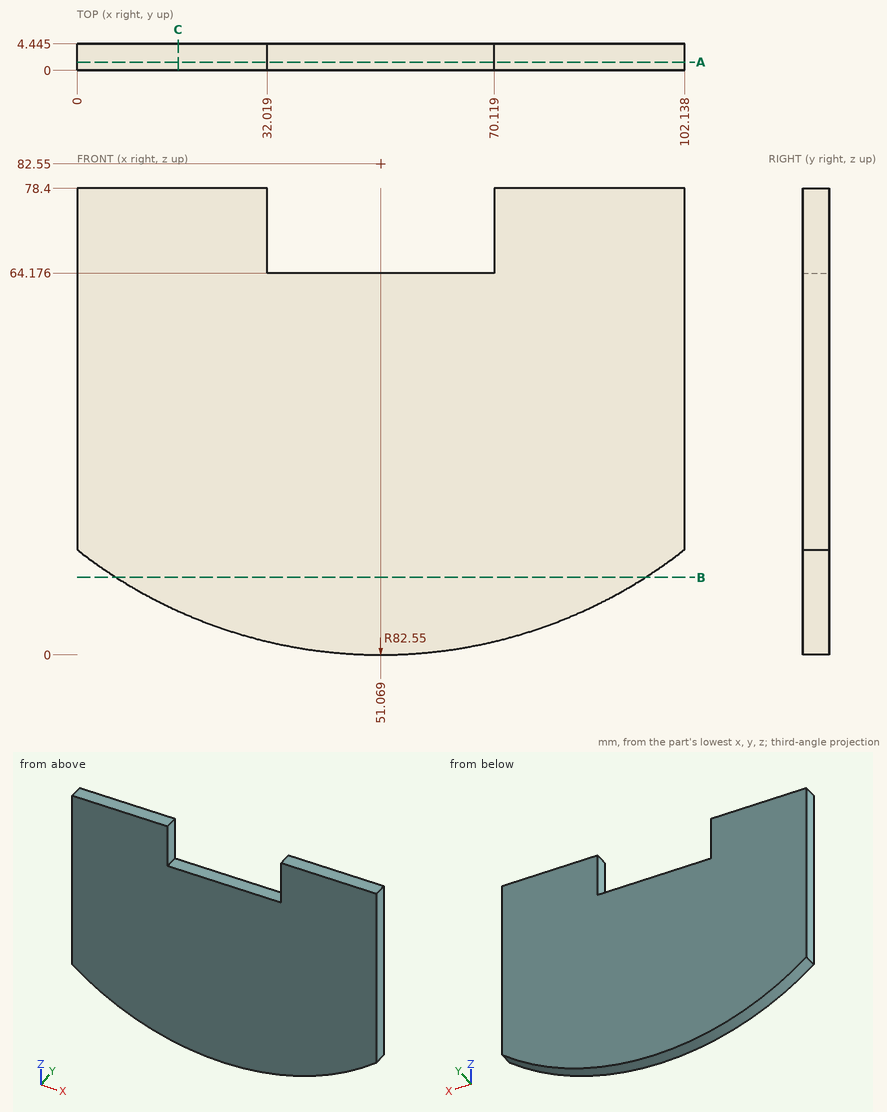
Source: three-view drawing plus pictorial views. Frame: mm from the lowest corner of the part. Round coordinates to 2 decimals unless told otherwise and drop trailing zeros. Order: outer loops, then holes, each group sorted by start corner. A loop starts at its lowest first (then second) coordinate and runs counter-clockwise, first axis right, second up. Notation, with made-up numbers: (16.25, 87) -> (54.25, 87) arc R32 cw to (54.25, 123) -> close; hole circle Ø9 at (38.5, 22). An arc over 180 degrees is marked (long way). Use one line per item in the form item = value.
(1) Section B-B on z = 13. Return loops of the section in (x, y) (1 decimal), and give its area (3 significant figures).
Results list:
outline = (6.6, 0) -> (95.5, 0) -> (95.5, 4.4) -> (6.6, 4.4) -> close
area = 395 mm^2
(2) Section A-A on y = 1.4. Return loops of the section in (x, z).
Results list:
outline = (0, 17.69) arc R82.55 ccw to (102.14, 17.69) -> (102.14, 78.4) -> (70.12, 78.4) -> (70.12, 64.18) -> (32.02, 64.18) -> (32.02, 78.4) -> (0, 78.4) -> close
(3) Ray query, probe 1 along X at (y, z) = (3.7, 64.5); probe 2 along Z at (x, y) = (50, 0.85); probe 3 along Z at (x, y) = (67.5, 2.5). Return the intervals inside material, ascending. Write a range as [from, to].
Results list:
probe_1 = [0, 32.02], [70.12, 102.14]
probe_2 = [0.01, 64.18]
probe_3 = [1.65, 64.18]
(4) Section C-C on x = 17. Return loops of the section in (y, z) (1 decimal), and give its area (3 significant figures).
Results list:
outline = (0, 7.4) -> (4.4, 7.4) -> (4.4, 78.4) -> (0, 78.4) -> close
area = 316 mm^2
(5) First-contact query: pin 1 Ø2 at (x, y) = (59.5, 2.5) entering from +Z; pin 2 Ø1 at (x, y) = (19, 3.5) entering from -Z (1 decimal). Flat tips, straight axial feed; report the tip coordinate or a pass-through.
Results list:
pin_1 = 64.18
pin_2 = 6.3
